```python
from build123d import *

# Parameters (mm, degrees)
SKETCH1_W           = 40
SKETCH1_H           = 40
BOSS_EXTRUDE1_DEPTH = 10
SKETCH2_R           = 18
SKETCH2_R_2         = 15
BOSS_EXTRUDE2_DEPTH = 60


with BuildPart() as part:
    # Sketch1 → Boss-Extrude1 (new body)
    with BuildSketch(Plane(origin=(0, 0, 0), x_dir=(1, 0, 0), z_dir=(0, 1, 0))):
        with Locations((20, -20)):
            Rectangle(SKETCH1_W, SKETCH1_H)
    extrude(amount=BOSS_EXTRUDE1_DEPTH)

    # Sketch2 → Boss-Extrude2 (add)
    with BuildSketch(Plane(origin=(0, 10, 0), x_dir=(1, 0, 0), z_dir=(0, 1, 0))):
        with Locations(Location((20, -20, 0), (0, 0, 270))):
            Circle(SKETCH2_R)
        with Locations(Location((20, -20, 0), (0, 0, 270))):
            Circle(SKETCH2_R_2, mode=Mode.SUBTRACT)
    extrude(amount=BOSS_EXTRUDE2_DEPTH)


solid = part.part
```
For this review, take the finished solid that the model builds, in its own axes (mm). A direction names the side the tool comes from. Coordinates: 2 decimals unless noted, no trailing zeros. Loops run counter-clockwise (first coordinate to the right, second up) from the corner with the lowest first, then second, coordinate; pieces in that order, holes last.
1. For faces 1 (the flat face through (40, 5, 20)), 2 (the flat face through (15, 10, 2)), list the 3-axis set-ups (+Z, -Z, +X, -X, +Y, -Y) from which the entire face can be reached by the end or side of a thin tool; tool diameter is ignored.
2. For line 1 (X direction, y = 22, z = 20); line 2 (X direction, y = 38, z = 28); line 3 (Z direction, x = 6.5, y = 56), list the stretches that pass through material, from the lowest coordinate up.
3. Insertion check: P1, Ø4, axis at y = 45, z = 10.5, coming from the -X side; P2, Ø8, axis at x = 17, y = 56.5, coming from the +Z side; P3, Ø5, axis at y = 13.5, z = 18.5, coming from the -X side. Each pin has a flat end and moves straight along its axis. Give the tip position at first contact, or say it passes through.
4. Mouldability with a two-part tool opening along Z and no side actions: class faces 3 (the flat face through (35, 70, 16)), 4 (the cylindrical face through (5.357, 39.58, 16.748)), 5 (the cylindrical face through (4.031, 39.58, 28.306)), 6 (the flat face through (20, 10, 20)) as +Z half, -Z half, draft (parallel to the pull), parting line (faces both ways), or undercut.
5. Add section A-A, the plane x = 20. Give the boundary of the cut face in (y, z), then the cut area to 3 significant figures.
6. Add section C-C, the plane y = 13. Give the boundary of the cut face in (x, z).
7. Add section B-B, the plane z = 36.5. Give the boundary of the cut face in (x, y), then the cut area to 3 significant figures.
8. Add section D-D, the plane z = 20. Give the boundary of the cut face in (x, y).
Result:
1. face 1: +Z, -Z, +X, +Y, -Y
1. face 2: +Y
2. line 1: x = 2 to 5, 35 to 38
2. line 2: x = 3.88 to 7.31, 32.69 to 36.12
2. line 3: z = 8.09 to 13.46, 26.54 to 31.91
3. P1: stops at x = 3.64
3. P2: stops at z = 38
3. P3: stops at x = 2
4. face 3: draft
4. face 4: undercut
4. face 5: parting line
4. face 6: undercut
5. outline: (0, 0) - (10, 0) - (10, 2) - (70, 2) - (70, 5) - (10, 5) - (10, 35) - (70, 35) - (70, 38) - (10, 38) - (10, 40) - (0, 40) - close
5. area: 760 mm2
6. outline: circle Ø36 at (20, 20); hole circle Ø30 at (20, 20)
7. outline: (0, 0) - (40, 0) - (40, 10) - (27.19, 10) - (27.19, 70) - (12.81, 70) - (12.81, 10) - (0, 10) - close
7. area: 1,260 mm2
8. outline: (0, 0) - (40, 0) - (40, 10) - (38, 10) - (38, 70) - (35, 70) - (35, 10) - (5, 10) - (5, 70) - (2, 70) - (2, 10) - (0, 10) - close
